For this review, use the dimensioned drawing (mm, ordinates from the lowest corner) and the shaded views. A direction names the side the tool comes from. Round coordinates to 2 decimals unless told otherwise and drop trailing zeros. Loops run counter-clockwise (first coordinate to the right, second up) from the corner with the lowest first, then second, coordinate; pieces in that order, holes last. Notation, with made-up numbers: M 13,-17 L 27,-17 A29 ccw 27,4 Z; hole C 16.5,1 d8. An arc over 180 degrees is marked long. Answer as a JSON object with one key per item and string values. Group by question number.
Item 1: Consider section D-D (x = 20). Give the boundary of the cut face in (y, z).
Item 2: The part is to be moulded in two halves that separate along Y. For the marked faces 4, 5, 6 and 7, say which applies: +Y half, -Y half, draft (parallel to the pull), parting line (faces both ways), or undercut.
Item 3: Consider section B-B (x = 16.75). Give the boundary of the cut face in (y, z).
Item 4: Tool access review of the marked faces 1, 2 and 3: name each direction out of +Z, -Z, +X, -X, +Y, -Y from which nothing blocks a thin tool from reaching the whole face with its end or side.
Item 5: Insertion check: P1, Ø9.5, axis at x = 12.7, y = 11, coming from the -Z side; P2, Ø1.5, axis at y = 17.5, z = 8, coming from the -X side; P3, Ø10, axis at x = 14, z = 28, coming from the +Y side. Each pin has a flat end and moves straight along its axis. Give the tip position at first contact, or say it passes through.
Item 6: To check wall thickness, follow line 1 (Y direction, x = 13, z = 33) (1 decimal); line 2 (X direction, y = 9.5, z = 29) (1 decimal); line 3 (Z direction, x = 13.75, y = 10). State the ranges of each line that lie inside material, in increasing order.
Item 7: Consider section A-A (y = 5.75). Give the boundary of the cut face in (x, z).
Item 8: Consider section C-C (z = 13). Give the boundary of the cut face in (x, y), and give its area (3 significant figures).
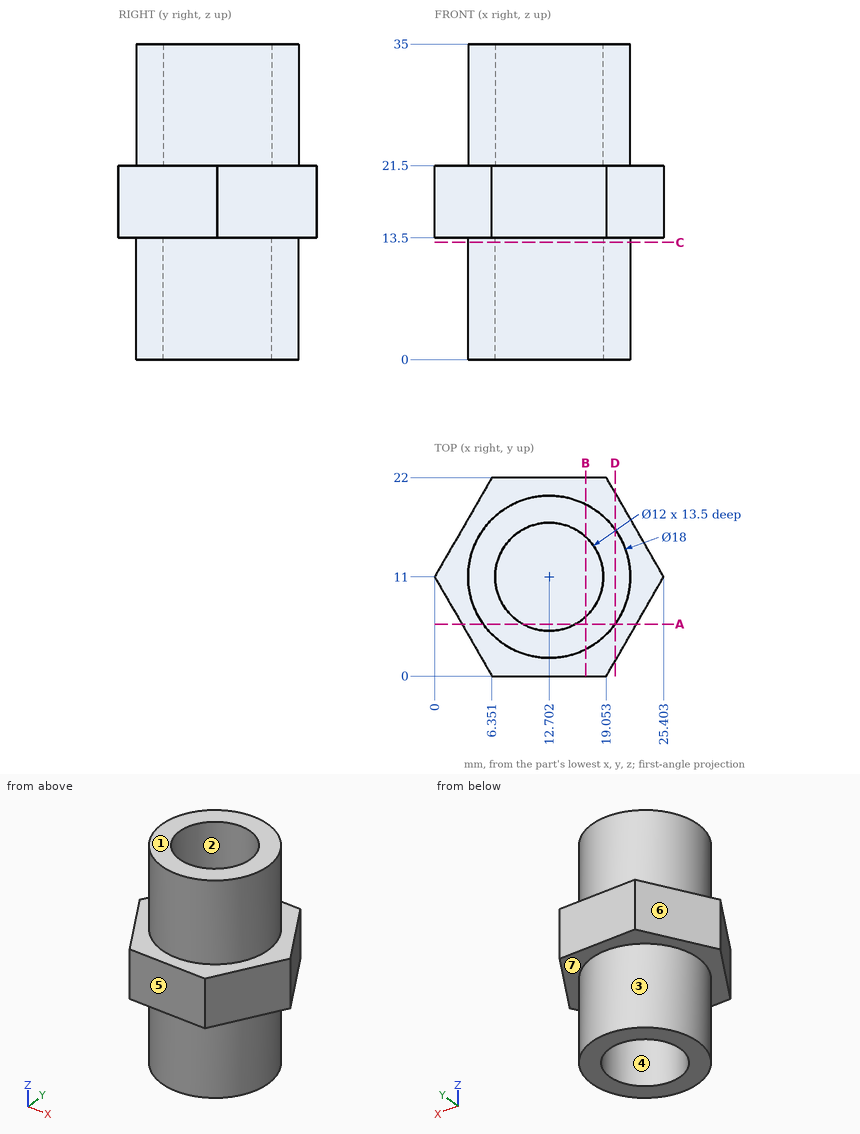
Geometry results:
{
 "1": {"outline": "M 1.64,13.5 L 5.73,13.5 L 5.73,0 L 16.27,0 L 16.27,13.5 L 20.36,13.5 L 20.36,21.5 L 16.27,21.5 L 16.27,35 L 5.73,35 L 5.73,21.5 L 1.64,21.5 Z"},
 "2": {"face 4": "undercut", "face 5": "-Y half", "face 6": "+Y half", "face 7": "draft"},
 "3": {"outline": "M 0,13.5 L 2.96,13.5 L 2.96,0 L 6.57,0 L 6.57,13.5 L 15.43,13.5 L 15.43,0 L 19.04,0 L 19.04,13.5 L 22,13.5 L 22,21.5 L 19.04,21.5 L 19.04,35 L 15.43,35 L 15.43,21.5 L 6.57,21.5 L 6.57,35 L 2.96,35 L 2.96,21.5 L 0,21.5 Z"},
 "4": {"face 1": "+Z, +X, -X, +Y, -Y", "face 2": "+Z", "face 3": "-Z"},
 "5": {"P1": "stops at z = 13.5", "P2": "stops at x = 5.78", "P3": "stops at y = 20"},
 "6": {"line 1": "y = 2 to 5, 17 to 20", "line 2": "x = 3.8 to 6.9, 18.5 to 21.6", "line 3": "z = 13.5 to 21.5"},
 "7": {"outline": "M 3.03,13.5 L 5.39,13.5 L 5.39,0 L 9.8,0 L 9.8,13.5 L 15.61,13.5 L 15.61,0 L 20.01,0 L 20.01,13.5 L 22.37,13.5 L 22.37,21.5 L 20.01,21.5 L 20.01,35 L 15.61,35 L 15.61,21.5 L 9.8,21.5 L 9.8,35 L 5.39,35 L 5.39,21.5 L 3.03,21.5 Z"},
 "8": {"outline": "C 12.7,11 d18; hole C 12.7,11 d12", "area": "141 mm^2"}
}
